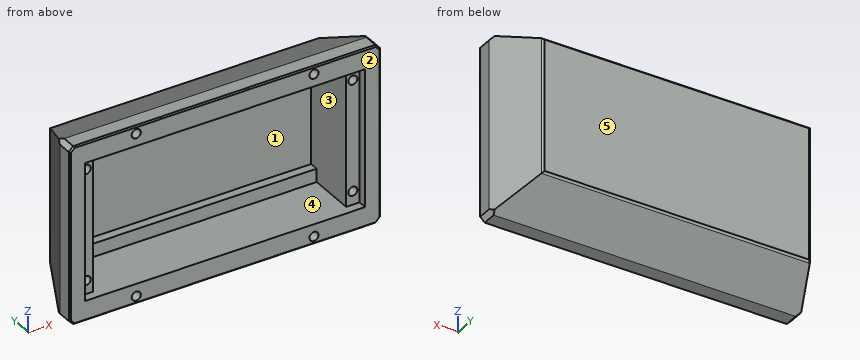
```python
from build123d import *
from OCP.BRepFilletAPI import BRepFilletAPI_MakeChamfer

# Parameters (mm, degrees)
SKETCH1_W           = 140
SKETCH1_H           = 80
BOSS_EXTRUDE1_DEPTH = 7
CHAMFER1_SIZE       = 2
SKETCH4_R           = 2.05
CUT_EXTRUDE1_DEPTH  = 7
SKETCH5_W           = 114
SKETCH5_H           = 50
CUT_EXTRUDE2_DEPTH  = 29
SKETCH6_W           = 114
SKETCH6_H           = 62
CUT_EXTRUDE3_DEPTH  = 25
SKETCH7_W           = 6
SKETCH7_H           = 62
CUT_EXTRUDE4_DEPTH  = 4
SKETCH8_R           = 2.05
CUT_EXTRUDE5_DEPTH  = 6
CHAMFER2_SIZE       = 1
CHAMFER2_SIZE2      = 0.471497246
CHAMFER3_SIZE       = 0.6


with BuildPart() as part:
    # Sketch1 → Boss-Extrude1 (new body)
    with BuildSketch(Plane(origin=(0, 0, 0), x_dir=(1, 0, 0), z_dir=(0, 1, 0))):
        Rectangle(SKETCH1_W, SKETCH1_H)
    extrude(amount=BOSS_EXTRUDE1_DEPTH)

    # Sketch3 → Loft2 section 0
    with BuildSketch(Plane(origin=(0, 7, 0), x_dir=(1, 0, 0), z_dir=(0, 1, 0))):
        with BuildLine():
            Line((70, -40), (70, 40))
            Line((70, 40), (-70, 40))
            Line((-70, 40), (-70, -40))
            Line((-70, -40), (70, -40))
        make_face()
    # Sketch2 → Loft2 section 1
    with BuildSketch(Plane(origin=(0, 30, 0), x_dir=(1, 0, 0), z_dir=(0, 1, 0))):
        with BuildLine():
            Line((-60, -30), (60, -30))
            Line((60, -30), (60, 30))
            Line((60, 30), (-60, 30))
            Line((-60, 30), (-60, -30))
        make_face()
    loft()

    # Chamfer1
    chamfer1_edges = [part.edges().sort_by_distance(p)[0] for p in [
        (-70, 3.5, 40),
        (70, 3.5, 40),
        (70, 3.5, -40),
        (-70, 3.5, -40),
    ]]
    chamfer(chamfer1_edges, length=CHAMFER1_SIZE)

    # Sketch4 → Cut-Extrude1 (cut)
    with BuildSketch(Plane.XZ):
        with Locations(Location((40, -36.5, 0), (0, 0, 270))):
            Circle(SKETCH4_R)
        with Locations(Location((-40, -36.5, 0), (0, 0, 270))):
            Circle(SKETCH4_R)
    cut_extrude1 = extrude(amount=-CUT_EXTRUDE1_DEPTH, mode=Mode.SUBTRACT)

    # Sketch5 → Cut-Extrude2 (cut)
    with BuildSketch(Plane.XZ):
        Rectangle(SKETCH5_W, SKETCH5_H)
    extrude(amount=-CUT_EXTRUDE2_DEPTH, mode=Mode.SUBTRACT)

    # Mirror1: Cut-Extrude1 across plane
    add(cut_extrude1.mirror(Plane.XY), mode=Mode.SUBTRACT)

    # Sketch6 → Cut-Extrude3 (cut)
    with BuildSketch(Plane.XZ):
        Rectangle(SKETCH6_W, SKETCH6_H)
    extrude(amount=-CUT_EXTRUDE3_DEPTH, mode=Mode.SUBTRACT)

    # Sketch7 → Cut-Extrude4 (cut)
    with BuildSketch(Plane.XZ):
        with Locations((-60, 0)):
            Rectangle(SKETCH7_W, SKETCH7_H)
        with Locations((60, 0)):
            Rectangle(SKETCH7_W, SKETCH7_H)
    extrude(amount=-CUT_EXTRUDE4_DEPTH, mode=Mode.SUBTRACT)

    # Sketch8 → Cut-Extrude5 (cut)
    with BuildSketch(Plane.XZ.offset(-4)):
        with Locations(Location((-60, 25, 0), (0, 0, 270))):
            Circle(SKETCH8_R)
        with Locations(Location((-60, -25, 0), (0, 0, 270))):
            Circle(SKETCH8_R)
        with Locations(Location((60, -25, 0), (0, 0, 90))):
            Circle(SKETCH8_R)
        with Locations(Location((60, 25, 0), (0, 0, 90))):
            Circle(SKETCH8_R)
    extrude(amount=-CUT_EXTRUDE5_DEPTH, mode=Mode.SUBTRACT)

    # Chamfer2: one chamfer whose edges measure the first distance from different faces: ONE call of the kernel's chamfer builder (chamfer() names one face for all edges)
    chamfer2_edges_1 = [part.edges().sort_by_distance(p)[0] for p in [
        (60, 30, 0),
    ]]
    chamfer2_side_1 = [part.faces().sort_by_distance(p)[0] for p in [
        (65.225405922, 17.98156638, 0),
    ]]
    chamfer2_edges_2 = [part.edges().sort_by_distance(p)[0] for p in [
        (0, 30, -30),
    ]]
    chamfer2_side_2 = [part.faces().sort_by_distance(p)[0] for p in [
        (0, 18.221212121, -35.121212121),
    ]]
    chamfer2_edges_3 = [part.edges().sort_by_distance(p)[0] for p in [
        (-60, 30, 0),
    ]]
    chamfer2_side_3 = [part.faces().sort_by_distance(p)[0] for p in [
        (-65.225405922, 17.98156638, 0),
    ]]
    chamfer2_edges_4 = [part.edges().sort_by_distance(p)[0] for p in [
        (0, 30, 30),
    ]]
    chamfer2_side_4 = [part.faces().sort_by_distance(p)[0] for p in [
        (0, 18.221212121, 35.121212121),
    ]]
    chamfer2 = BRepFilletAPI_MakeChamfer(part.part.solid().wrapped)
    for e in chamfer2_edges_1:
        chamfer2.Add(CHAMFER2_SIZE, CHAMFER2_SIZE2, e.wrapped, chamfer2_side_1[0].wrapped)  # the first distance lies on this face
    for e in chamfer2_edges_2:
        chamfer2.Add(CHAMFER2_SIZE, CHAMFER2_SIZE2, e.wrapped, chamfer2_side_2[0].wrapped)  # the first distance lies on this face
    for e in chamfer2_edges_3:
        chamfer2.Add(CHAMFER2_SIZE, CHAMFER2_SIZE2, e.wrapped, chamfer2_side_3[0].wrapped)  # the first distance lies on this face
    for e in chamfer2_edges_4:
        chamfer2.Add(CHAMFER2_SIZE, CHAMFER2_SIZE2, e.wrapped, chamfer2_side_4[0].wrapped)  # the first distance lies on this face
    add(Compound.cast(chamfer2.Shape()), mode=Mode.REPLACE)

    # Chamfer3
    chamfer3_edges = [part.edges().sort_by_distance(p)[0] for p in [
        (0, 0, 40),
        (70, 0, 0),
        (-70, 0, 0),
        (0, 0, -40),
        (-69, 0, -39),
        (69, 0, -39),
        (69, 0, 39),
        (-69, 0, 39),
    ]]
    chamfer(chamfer3_edges, length=CHAMFER3_SIZE)


solid = part.part
```
Design review of the part built by this model. Coordinates are the model's own, in mm. Face numbers are marked on the shaded views. A direction names the side the tool comes from. Give positions to 0.01 mm unless a question says otherwise; leave off trailing zeros. Write each loop counter-clockwise with the first axis right and the second up, starting at its lowest first coordinate (ties: lowest second). Pieces come first, ordered by that corner, then holes.
(1) Tool access review of the marked faces 4 and 5: name each direction out of +Z, -Z, +X, -X, +Y, -Y from which nothing blocks a thin tool from reaching the whole face with its end or side.
Checked values:
face 4: -Y
face 5: +Z, -Z, +X, -X, +Y
(2) Clearance check with flat-ended pins moving along their axes: pin 1 Ø1 at (y, z) = (22.5, -22.5) entering from +X; pin 2 Ø3.5 at (x, z) = (-39, -36) entering from -Y; pin 3 Ø5 at (x, z) = (-24.5, -2) entering from -Y; pin 4 Ø5 at (x, y) = (-28.5, 14) entering from +Z. State where each tip first meets the part, or that it passes through.
Checked values:
pin 1: stops at x = 63.48
pin 2: stops at y = 0
pin 3: stops at y = 29
pin 4: stops at z = 38.04
(3) Mouldability with a two-part tool opening along X and no side actions: class the marked faces 1, 2 and 3 as +X half, -X half, draft (parallel to the pull), parting line (faces both ways), or undercut.
Checked values:
face 1: undercut
face 2: draft
face 3: undercut
(4) Add section A-A (y = 2.5). Give the boundary of the cut face in (x, z).
Checked values:
outline: (-70, -38) - (-68, -40) - (68, -40) - (70, -38) - (70, 38) - (68, 40) - (-68, 40) - (-70, 38) - close; hole (-63, -31) - (63, -31) - (63, 31) - (-63, 31) - close; hole circle Ø4.1 at (-40, -36.5); hole circle Ø4.1 at (-40, 36.5); hole circle Ø4.1 at (40, -36.5); hole circle Ø4.1 at (40, 36.5)
(5) Wall thickness on line 1 along X through (y, z) = (6.6, -25); line 2 along X through (y, z) = (2, 36.5); line 3 along X through (y, z) = (8, 25): over which ranges is each line inside the solid? List them lowest first.
Checked values:
line 1: x = -70 to -62.05, -57.95 to -57, 57 to 57.95, 62.05 to 70
line 2: x = -70 to -42.05, -37.95 to 37.95, 42.05 to 70
line 3: x = -69.57 to -62.05, -57.95 to -57, 57 to 57.95, 62.05 to 69.57
